from build123d import *

# Parameters (mm, degrees)
F0_R     = 6.35
F1_DEPTH = 25.4


with BuildPart() as f1:
    # F0 (on Top) → F1 (new body, symmetric)
    with BuildSketch(Plane.XY):
        with BuildLine():
            Line((-12.661204, 44.061287), (-38.1, 0))
            Line((-38.1, 0), (38.1, 0))
            Line((38.1, 0), (12.661204, 44.061287))
            ThreePointArc((12.661204, 44.061287), (0, 51.371237), (-12.661204, 44.061287))
        make_face()
        with Locations((0, 36.751337)):
            Circle(F0_R, mode=Mode.SUBTRACT)
    extrude(amount=F1_DEPTH, both=True)


solid = f1.part
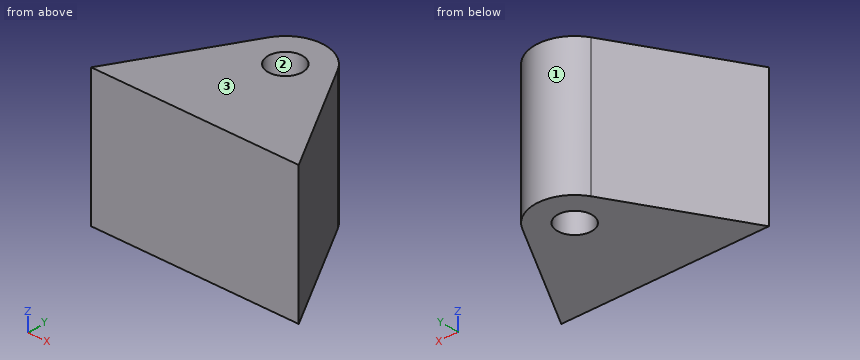
Geometry: final body of the model. Coordinates: model frame, mm. Face numbers are marked on the shaded views. Round coordinates to 2 decimals unless told otherwise and drop trailing zeros. Loops run counter-clockwise (first coordinate to the right, second up) from the corner with the lowest first, then second, coordinate; pieces in that order, holes last.
Q1. Section D-D on y = 12. Return loops of the section in (x, z), plus the area to 3 significant figures.
Q2. Section A-A on x = 0. Return loops of the section in (y, z), plus the area to 3 significant figures.
Q3. Pin query (flat end, axial travel): P1, Ø6, axis at x = -10, z = 3, coming from the -Y side; P2, Ø2, axis at y = 13.5, z = 13.5, coming from the +X side; P3, Ø2, axis at y = 32, z = -7, coming from the +X side; P4, Ø3, axis at x = -28, z = 13.5, coming from the +Y side. Return the tip coordinate at first contact, or that it passes through.
Q4. Section C-C on z = -19. Return loops of the section in (x, y), plus the area to 3 significant figures.
Q5. Material intervals for L1, parallel to X at y = 31, z = 4; L2, parallel to Y at x = 30, z = -16; L3, parallel to X at y = 6.5, z = 6, sorted ascending.
Q6. Section B-B on y = 34. Return loops of the section in (x, z).
Q7. Pull-direction query (X, two-part tool) for the marked faces 1, 2 and 3; classes: released by +X, released by -X, zero draft, split by the parting line, or undercut.
Evaluation:
1. outline: (-31.17, -25.4) - (31.17, -25.4) - (31.17, 25.4) - (-31.17, 25.4) - close
1. area: 3,170 mm2
2. outline: (0, -25.4) - (30.4, -25.4) - (30.4, 25.4) - (0, 25.4) - close; (43.1, -25.4) - (51.37, -25.4) - (51.37, 25.4) - (43.1, 25.4) - close
2. area: 1,960 mm2
3. P1: stops at y = 0
3. P2: stops at x = 30.88
3. P3: stops at x = 20.2
3. P4: stops at y = 20.09
4. outline: (-38.1, 0) - (38.1, 0) - (12.66, 44.06) arc R14.62 ccw to (-12.66, 44.06) - close; hole circle Ø12.7 at (0, 36.75)
4. area: 2,240 mm2
5. L1: x = -20.2 to -2.69, 2.69 to 20.2
5. L2: y = 0 to 14.03
5. L3: x = -34.35 to 34.35
6. outline: (-18.47, -25.4) - (-5.72, -25.4) - (-5.72, 25.4) - (-18.47, 25.4) - close; (5.72, -25.4) - (18.47, -25.4) - (18.47, 25.4) - (5.72, 25.4) - close
7. face 1: split by the parting line
7. face 2: undercut
7. face 3: zero draft
